```python
from build123d import *

# Parameters (mm, degrees)
SKETCH2_R           = 2.4892
BOSS_EXTRUDE1_DEPTH = 1.5875


with BuildPart() as part:
    # Sketch2 → Boss-Extrude1 (new body)
    with BuildSketch(Plane(origin=(-406.836680709, 67.862442728, -60.114831645), x_dir=(-0.15204147849631244, -0.03655570855361372, 0.9876978632095945), z_dir=(0.9760593070661704, -0.16281169315785926, 0.1442240675496927))):
        with BuildLine():
            Line((-544.785785419, 305.655391385), (-546.457439277, 275.221266239))
            ThreePointArc((-546.457439277, 275.221266239), (-537.469166999, 265.1882103), (-527.436111061, 274.176482578))
            Line((-527.436111061, 274.176482578), (-525.764457203, 304.610607723))
            Line((-525.764457203, 304.610607723), (-544.785785419, 305.655391385))
        make_face()
        with Locations(Location((-536.946775169, 274.698874408, 0), (0, 0, 86.498585174))):
            Circle(SKETCH2_R, mode=Mode.SUBTRACT)
    extrude(amount=BOSS_EXTRUDE1_DEPTH)


with BuildPart() as body_2:
    # Mirror2: mirrored copy
    add(part.part.mirror(Plane(origin=(0, 0, 0), x_dir=(0, 0, 1), z_dir=(1, 0, 0))))


solid = body_2.part
```
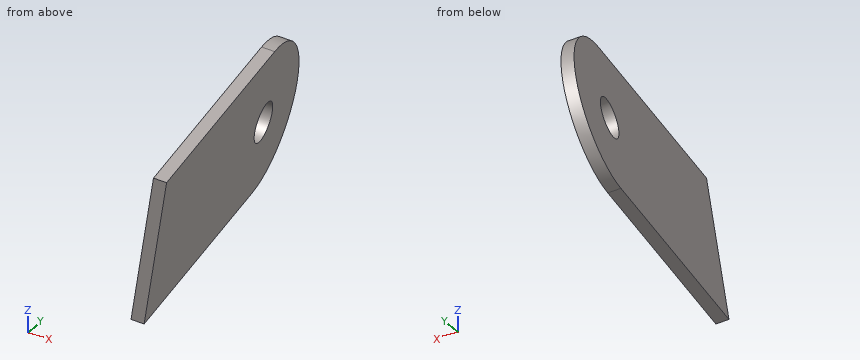
Can you work these out from the model? Positions are in its coordinate system, mm. Round coordinates to 2 decimals unless told otherwise and drop trailing zeros. Loops run counter-clockwise (first coordinate to the right, second up) from the corner with the lowest first, then second, coordinate; pieces in that order, holes last.
Item 1: Please list where these lines run through material, in increasing order: L1, parallel to X at y = -206, z = -604.5; L2, parallel to X at y = -187, z = -611.25.
Item 2: Suppose I cut it at B-B, the plane y = -209.5. Write out the boundary of the cut face in (x, z), then the cut area to 3 significant figures.
Item 3: Suppose I cut it at A-A, the plane x = 371. Write out the boundary of the cut face in (y, z), then the cut area to 3 significant figures.
Item 4: Will these pins go through, and if not, where does the flat tip stop? pin 1 Ø1.5 at (y, z) = (-195, -599.5) entering from -X; pin 2 Ø8 at (y, z) = (-180.5, -605) entering from +X; pin 3 Ø5 at (x, z) = (367, -612) entering from +Y.
Reported:
1. L1: x = 370.45 to 372.08
1. L2: x = 366.29 to 367.91
2. outline: (369.28, -616.41) - (370.87, -616.65) - (373.65, -597.8) - (372.06, -597.57) - close
2. area: 30.7 mm2
3. outline: (-213.73, -609.52) - (-213.68, -616.59) - (-210.29, -616.65) - (-193.5, -597.7) - (-203.1, -597.53) - close
3. area: 163 mm2
4. pin 1: stops at x = 369.19
4. pin 2: stops at x = 368.64
4. pin 3: stops at y = -174.4
